Geometry check sheet. Reference: the model listing, model coordinates, mm. Round coordinates to 2 decimals unless told otherwise and drop trailing zeros. Write each loop counter-clockwise with the first axis right and the second up, starting at its lowest first coordinate (ties: lowest second). Pieces come first, ordered by that corner, then holes. Notation, with made-up numbers: M 78.5,4.5 L 87.5,4.5 A22 ccw 87.5,42.5 Z; hole C 41,23 d11. An arc over 180 degrees is marked long. One line per item, written item: value. Start each with the question number.
1. Scan lines: probe 1 along Y at (x, z) = (0.4, 16); probe 2 along X at (y, z) = (4.25, 36); probe 3 along X at (y, z) = (-6.5, 20.5). Record each from-to range of solid material in increasing order. Write a range as [from, to].
2. Section check C-C (y = -6.5). Record the boundary of the cut face in (x, z), and give its area (3 significant figures).
3. Section check A-A (z = 14). Record the boundary of the cut face in (x, y) (3 decimals).
4. Section check B-B (x = 0.1). Record the boundary of the cut face in (y, z).
from build123d import *

# Parameters (mm, degrees)
F1_DEPTH    = 40.64
F2_T1_DEPTH = 62.6370452561
F3_T1_DEPTH = 52.9367221242


# Not quite as in the source:
# - a fillet or chamfer that OpenCascade refuses, or shapes differently, is made with other operations: its cross-section is extruded or revolved along the edge and cut away or added


with BuildPart() as f1:
    # F0 (on Top) → F1 (new body)
    with BuildSketch(Plane.XY):
        with BuildLine():
            Line((0.635, -8.255), (1.27, -8.255))
            Line((1.27, -8.255), (1.27, 8.255))
            Line((1.27, 8.255), (-1.27, 8.255))
            Line((-1.27, 8.255), (-1.27, -8.255))
            Line((-1.27, -8.255), (-0.635, -8.255))
            ThreePointArc((-0.635, -8.255), (0, -7.62), (0.635, -8.255))
        make_face()
        with BuildLine():
            ThreePointArc((-0.635, -8.255), (0, -8.89), (0.635, -8.255))
            Line((0.635, -8.255), (-0.635, -8.255))
        make_face()
        with BuildLine():
            Line((-0.635, -8.255), (0.635, -8.255))
            ThreePointArc((0.635, -8.255), (0, -7.62), (-0.635, -8.255))
        make_face()
    extrude(amount=F1_DEPTH)

    # F2: fillet of radius 5.08 on 1 edges, made by hand

    # F2_s2 → F2_t1 (cut)
    with BuildSketch(Plane.XY.offset(-10.9985226281)):
        with BuildLine():
            ThreePointArc((1.27, 8.255), (-0.5894090512, 6.3955909488), (-1.27, 3.8555909488))
            Line((-1.27, 3.8555909488), (-1.27, 8.255))
            Line((-1.27, 8.255), (1.27, 8.255))
        make_face()
    extrude(amount=F2_T1_DEPTH, mode=Mode.SUBTRACT)

    # F3: fillet of radius 5.08 on 2 edges, made by hand

    # F3_s2 → F3_t1 (cut)
    with BuildSketch(Plane.XY.offset(-6.1483610621)):
        with BuildLine():
            ThreePointArc((-0.635, -8.255), (-1.1086888497, -7.0656555752), (-1.27, -5.7956555752))
            Line((-1.27, -5.7956555752), (-1.27, -8.255))
            Line((-1.27, -8.255), (-0.635, -8.255))
        make_face()
        with BuildLine():
            ThreePointArc((0.635, -8.255), (1.1086888497, -7.0656555752), (1.27, -5.7956555752))
            Line((1.27, -5.7956555752), (1.27, -8.255))
            Line((1.27, -8.255), (0.635, -8.255))
        make_face()
    extrude(amount=F3_T1_DEPTH, mode=Mode.SUBTRACT)


solid = f1.part
Result sheet:
1. probe 1: y = [-8.75, 7.62]
1. probe 2: x = [-1.25, 1.27]
1. probe 3: x = [-1.22, 1.22]
2. outline: M -1.22,0 L 1.22,0 L 1.22,40.64 L -1.22,40.64 Z
2. area: 99.2 mm2
3. outline: M -1.27,-5.796 A5.08 ccw -0.635,-8.255 A0.635 ccw 0.635,-8.255 A5.08 ccw 1.27,-5.796 L 1.27,8.255 A5.08 ccw -1.27,3.856 Z
4. outline: M -8.88,0 L 7.33,0 L 7.33,40.64 L -8.88,40.64 Z
